Autodesk Fusion 360 part; units mm, degrees
sketch "Sketch1" plane through (0, 0, 0) normal (0, 0, 1) x (1, 0, 0)
  line L0 (-75, 150) -> (75, 150)
  line L1 (75, 150) -> (75, -150)
  line L2 (75, -150) -> (-75, -150)
  line L3 (-75, -150) -> (-75, 150)
  line L4 (-75, 150) -> (75, -150) construction
  line L5 (75, 150) -> (-75, -150) construction
  line L6 (50, 135) -> (-50, 135)
  line L7 (-50, 135) -> (-50, -135)
  line L8 (-50, -135) -> (50, -135)
  line L9 (50, -135) -> (50, 135)
  line L10 (50, 135) -> (-50, -135) construction
  line L11 (-50, 135) -> (50, -135) construction
  line L12 (-30, 135) -> (30, 135)
  line L13 (30, 135) -> (30, 130)
  line L14 (30, 130) -> (-30, 130)
  line L15 (-30, 130) -> (-30, 135)
  line L16 (-50, 40) -> (-45, 40)
  line L17 (-45, 40) -> (-45, -40)
  line L18 (-45, -40) -> (-50, -40)
  line L19 (-50, -40) -> (-50, 40)
  line L20 (-30, -135) -> (30, -135)
  line L21 (30, -135) -> (30, -130)
  line L22 (30, -130) -> (-30, -130)
  line L23 (-30, -130) -> (-30, -135)
  line L24 (50, 40) -> (45, 40)
  line L25 (45, 40) -> (45, -40)
  line L26 (45, -40) -> (50, -40)
  line L27 (50, -40) -> (50, 40)
  line L28 (-50, -80) -> (-40, -80)
  line L29 (-40, -80) -> (-40, -120)
  line L30 (-40, -120) -> (-50, -120)
  line L31 (-50, -120) -> (-50, -80)
  line L32 (50, -120) -> (40, -120)
  line L33 (40, -120) -> (40, -80)
  line L34 (40, -80) -> (50, -80)
  line L35 (50, -80) -> (50, -120)
  line L36 (50, 120) -> (40, 120)
  line L37 (40, 120) -> (40, 80)
  line L38 (40, 80) -> (50, 80)
  line L39 (50, 80) -> (50, 120)
  line L40 (-50, 120) -> (-40, 120)
  line L41 (-40, 120) -> (-40, 80)
  line L42 (-40, 80) -> (-50, 80)
  line L43 (-50, 80) -> (-50, 120)
  dimension "d1" = 300
  dimension "d2" = 150
  dimension "d3" = 270
  dimension "d4" = 100
  dimension "d5" = 60
  dimension "d6" = 20
  dimension "d7" = 5
  dimension "d8" = 80
  dimension "d9" = 95
  dimension "d10" = 5
  dimension "d11" = 60
  dimension "d12" = 5
  dimension "d13" = 20
  dimension "d14" = 80
  dimension "d15" = 5
  dimension "d16" = 95
  dimension "d19" = 10
  dimension "d20" = 40
  dimension "d21" = 40
  dimension "d22" = 10
  dimension "d23" = 40
  dimension "d24" = 40
  dimension "d25" = 10
  dimension "d26" = 40
  dimension "d27" = 40
  dimension "d28" = 10
  dimension "d29" = 40
  dimension "d30" = 40
extrude "Extrude2" add sketch "Sketch1" along normal blind 4 contours L0 L1 L2 L3 | L6 L12 L13 L14 L15 | L9 L36 L37 L38 L39 | L9 L24 L25 L26 L27 | L7 L40 L41 L42 L43 | L9 L32 L33 L34 L35 | L7 L16 L17 L18 L19 | L7 L28 L29 L30 L31
sketch "Sketch2" plane through (0, 0, 0) normal (0, 0, 1) x (1, 0, 0)
  line L0 (0, 0) -> (-57, 0) construction
  circle A0 centre (-57, 0) radius 2
  line L1 (0, 0) -> (57, 0) construction
  circle A1 centre (57, 0) radius 2
  line L2 (0, 0) -> (0, -99) construction
  line L3 (0, -99) -> (-50, -99) construction
  line L4 (0, -99) -> (50, -99) construction
  line L5 (0, 0) -> (0, 99) construction
  line L6 (0, 99) -> (50, 99) construction
  line L7 (0, 99) -> (-50, 99) construction
  circle A2 centre (50, 99) radius 2
  circle A3 centre (-50, 99) radius 2
  circle A4 centre (50, -99) radius 2
  circle A5 centre (-50, -99) radius 2
  dimension "d33" = 57
  dimension "d35" = 4
  dimension "d36" = 57
  dimension "d37" = 4
  dimension "d38" = 99
  dimension "d39" = 50
  dimension "d40" = 50
  dimension "d41" = 99
  dimension "d42" = 50
  dimension "d43" = 4
  dimension "d44" = 4
  dimension "d45" = 50
  dimension "d46" = 4
  dimension "d47" = 4
extrude "Extrude3" cut sketch "Sketch2" along normal through all
sketch "Sketch3" plane through (0, 0, 0) normal (0, 0, -1) x (1, 0, 0)
  circle A0 centre (57, 0) radius 2
  circle A1 centre (-50, 99) radius 2
  circle A2 centre (-50, -99) radius 2
  circle A3 centre (-57, 0) radius 2
  circle A4 centre (50, 99) radius 2
  circle A5 centre (50, -99) radius 2
  line L0 (50, -120) -> (50, -135)
  line L1 (50, -135) -> (30, -135)
  line L2 (30, -135) -> (30, -130)
  line L3 (30, -130) -> (-30, -130)
  line L4 (-30, -130) -> (-30, -135)
  line L5 (-30, -135) -> (-50, -135)
  line L6 (-50, -135) -> (-50, -120)
  line L7 (-50, -120) -> (-40, -120)
  line L8 (-40, -120) -> (-40, -80)
  line L9 (-40, -80) -> (-50, -80)
  line L10 (-50, -80) -> (-50, -40)
  line L11 (-50, -40) -> (-45, -40)
  line L12 (-45, -40) -> (-45, 40)
  line L13 (-45, 40) -> (-50, 40)
  line L14 (-50, 40) -> (-50, 80)
  line L15 (-50, 80) -> (-40, 80)
  line L16 (-40, 80) -> (-40, 120)
  line L17 (-40, 120) -> (-50, 120)
  line L18 (-50, 120) -> (-50, 135)
  line L19 (-50, 135) -> (50, 135)
  line L20 (50, 135) -> (50, 120)
  line L21 (50, 120) -> (40, 120)
  line L22 (40, 120) -> (40, 80)
  line L23 (40, 80) -> (50, 80)
  line L24 (50, 80) -> (50, 40)
  line L25 (50, 40) -> (45, 40)
  line L26 (45, 40) -> (45, -40)
  line L27 (45, -40) -> (50, -40)
  line L28 (50, -40) -> (50, -80)
  line L29 (50, -80) -> (40, -80)
  line L30 (40, -80) -> (40, -120)
  line L31 (40, -120) -> (50, -120)
  line L32 (75, 150) -> (-75, 150)
  line L33 (-75, 150) -> (-75, -150)
  line L34 (-75, -150) -> (75, -150)
  line L35 (75, -150) -> (75, 150)
The listing builds one solid part. Answer for the finished solid, in the listing's coordinates (mm). Coordinates: 2 decimals unless noted, no trailing zeros. Write each loop counter-clockwise with the first axis right and the second up, starting at its lowest first coordinate (ties: lowest second). Pieces come first, ordered by that corner, then holes. Notation, with made-up numbers: (26.5, 4.5) - (48.5, 4.5) arc R5 ccw to (48.5, 10.5) - close; hole circle Ø6 at (56.5, -10). An arc over 180 degrees is marked (long way). Answer as CSV lines item,"result".
1. Find section C-C (z = 1.8). Give the number of separate pieces and of enclosed holes in the cut face, plus the area to 3 significant figures.
Computed values:
separate pieces,"1"
enclosed holes,"7"
area,"20,600 mm²"
2. Straight lines are drawn through the part: line 1 (Y direction, x = -41, z = 3.8); line 2 (X direction, y = -99, z = 0.95); line 3 (X direction, y = -28, z = 1.1). For each, find the intervals that lie inside material, in ascending order. Write a range as [from, to].
Computed values:
line 1,"y = [-150, -135], [-120, -80], [80, 120], [135, 150]"
line 2,"x = [-75, -52], [-48, -40], [40, 48], [52, 75]"
line 3,"x = [-75, -45], [45, 75]"
3. Find section A-A (y = -89.5). Give the vertices of the cut face in (x, z), plus the area to 3 significant figures.
Computed values:
outline,"(-75, 0) - (-40, 0) - (-40, 4) - (-75, 4) - close; (40, 0) - (75, 0) - (75, 4) - (40, 4) - close"
area,"280 mm²"
4. Find section B-B (x = 16.5). Give the vertices of the cut face in (y, z).
Computed values:
outline,"(-150, 0) - (-135, 0) - (-135, 4) - (-150, 4) - close; (130, 0) - (150, 0) - (150, 4) - (130, 4) - close"
5. Given P1, Ø10, axis at x = 44, y = -60, coming from the -Z side; P2, Ø4.5, axis at x = 50, y = 99, coming from the -Z side, each flat-ended and moving along its own axis, determine where each tip first touches the part or whether it passes through.
Computed values:
P1,"passes through"
P2,"stops at z = 0"
